Answer from the drawing. Dimensions are ordinates in mm from the lowest x, y and z of the part. A direction names the side the tool comes from. Round coordinates to 2 decimals unless told otherwise and drop trailing zeros. Write each loop counter-clockwise with the first axis right and the second up, starting at its lowest first coordinate (ties: lowest second). Pieces come first, ordered by that corner, then holes. Notation, with made-up numbers: M 47,27.5 L 62,27.5 A22 cw 62,52.5 Z; hole C 50.5,-16.5 d1. An arc over 180 degrees is marked long. One line per item, written item: value. Start each with the question number.
(1) Section B-B (x = 12) is taken. Determine the outline of the cut face in (y, z) (1 decimal).
(2) For the marked faces 4, 5, 6 and 7, determine the directions among +Z, -Z, +X, -X, +Y, -Y from which every point of the face is accessible in a straight line to the end or side of a thin tool.
(3) Consider probe 1 along Z at (x, y) = (76, 3.5); probe 2 along X at (y, z) = (13, 76); probe 3 along Z at (x, y) = (109, 16.5) (1 decimal). Determine where each line is inside the solid, lowest interval first.
(4) For a pull along Z with two mould halves and no side action, classify the marked faces 1, 2 and 3 as released by +Z, released by -Z, zero draft, split by the parting line, or undercut.
(5) Section A-A (z = 76) is taken. Determine the outline of the cut face in (x, y), plus the area to 3 significant figures.
(6) Section C-C (x = 76) is taken. Determine the outline of the cut face in (y, z).
(7) Given P1, Ø7, axis at x = 87, y = 21, coming from the -Z side; P2, Ø12, axis at x = 124.5, y = 12, coming from the +Z side (1 decimal); P3, Ø8, axis at x = 107.5, y = 6, coming from the +Z side, each flat-ended and moving along its own axis, determine where each tip first touches the part or whether it passes through.
(8) Section D-D (z = 112) is taken. Determine the outline of the cut face in (x, y) (1 decimal), plus the area to 3 significant figures.
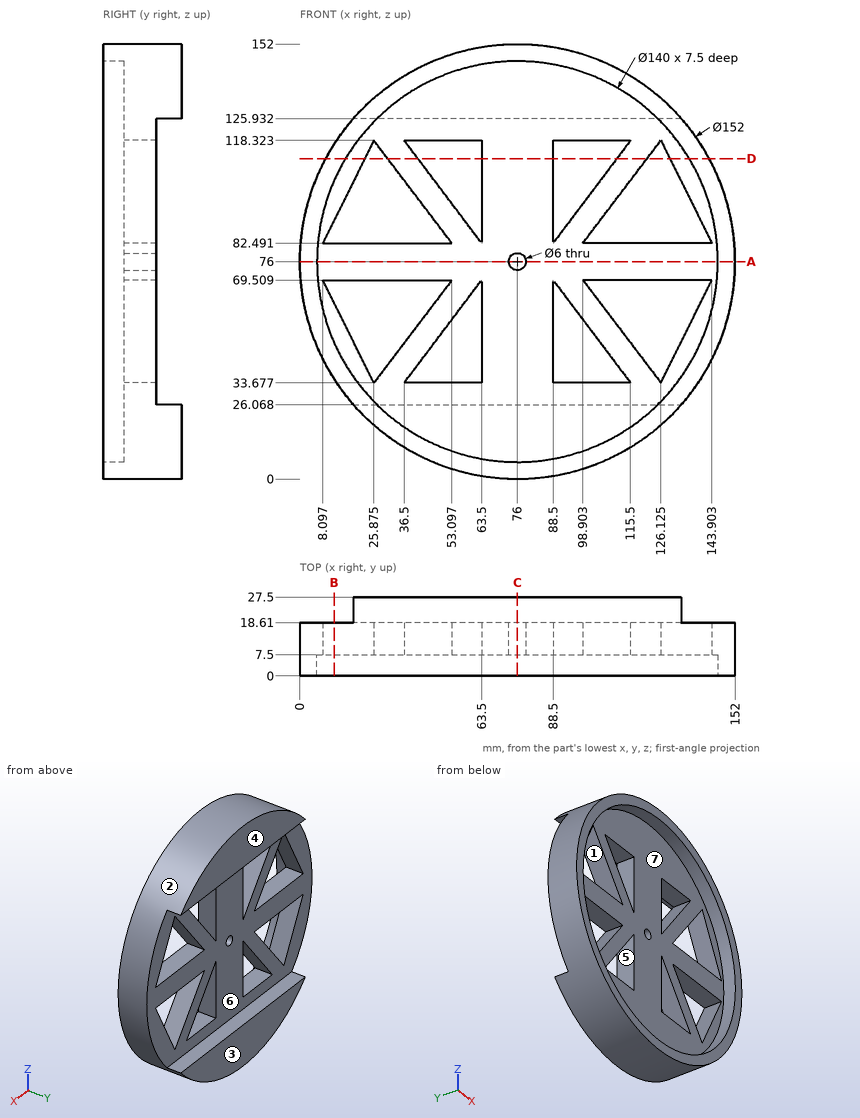
Recorded:
1. outline: M 0,35 L 18.6,35 L 18.6,61.6 L 7.5,61.6 L 7.5,47.6 L 0,47.6 Z; M 0,104.4 L 7.5,104.4 L 7.5,90.4 L 18.6,90.4 L 18.6,117 L 0,117 Z; M 7.5,69.5 L 18.6,69.5 L 18.6,82.5 L 7.5,82.5 Z
2. face 4: +Z, -Z, +X, -X, +Y
2. face 5: +Y, -Y
2. face 6: +X, -X, +Y
2. face 7: -Y
3. probe 1: z = 0 to 6, 146 to 152
3. probe 2: x = 0 to 73, 79 to 152
3. probe 3: z = 7.5 to 33.7, 42.3 to 56.2, 69.5 to 82.5, 95.8 to 109.7, 118.3 to 144.5
4. face 1: undercut
4. face 2: split by the parting line
4. face 3: zero draft
5. outline: M 0,0 L 6,0 L 6,7.5 L 73,7.5 L 73,18.61 L 0,18.61 Z; M 79,7.5 L 146,7.5 L 146,0 L 152,0 L 152,18.61 L 79,18.61 Z
5. area: 1,710 mm2
6. outline: M 0,0 L 27.5,0 L 27.5,26.07 L 18.61,26.07 L 18.61,73 L 7.5,73 L 7.5,6 L 0,6 Z; M 0,146 L 7.5,146 L 7.5,79 L 18.61,79 L 18.61,125.93 L 27.5,125.93 L 27.5,152 L 0,152 Z
7. P1: stops at z = 0.37
7. P2: stops at z = 139
7. P3: stops at z = 146.85
8. outline: M 9.1,0 L 16,0 L 16,7.5 L 22.7,7.5 L 22.7,18.6 L 9.1,18.6 Z; M 30.7,7.5 L 41.3,7.5 L 41.3,18.6 L 30.7,18.6 Z; M 63.5,7.5 L 88.5,7.5 L 88.5,18.6 L 63.5,18.6 Z; M 110.7,7.5 L 121.3,7.5 L 121.3,18.6 L 110.7,18.6 Z; M 129.3,7.5 L 136,7.5 L 136,0 L 142.9,0 L 142.9,18.6 L 129.3,18.6 Z
8. area: 920 mm2
